Verification items for this drawing (mm, ordinates from the low corner). A direction names the side the tool comes from. Coordinates: 2 decimals unless noted, no trailing zeros. Write each loop counter-clockwise with the first axis right and the second up, starting at its lowest first coordinate (ties: lowest second). Pieces come first, ordered by that corner, then holes. Notation, with made-up numbers: M 86.25,-15.75 L 98.25,-15.75 A7 ccw 98.25,-4.75 Z; hole C 89,-5.75 d11. An arc over 180 degrees is marked long. Write each question's results on one line, items separated by ' | '.
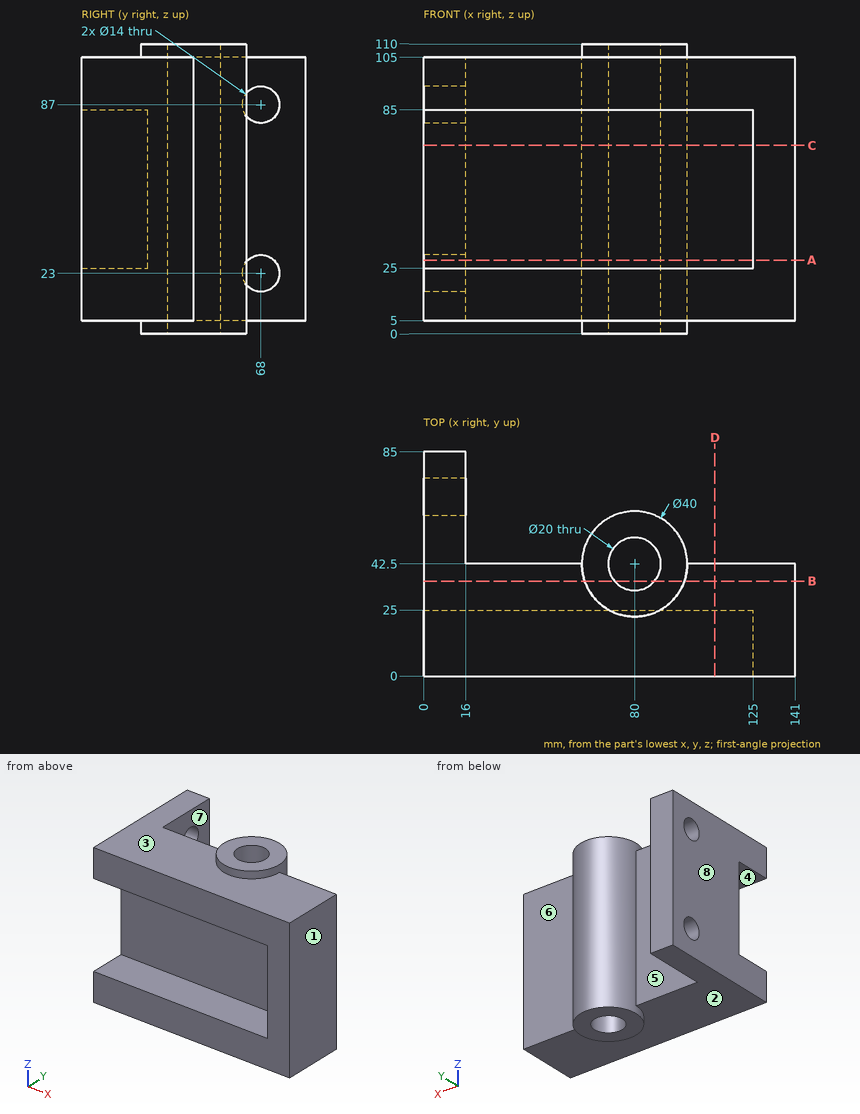
Q1. Sectioned sample at C-C on z = 71.5. Record the cut outline in (x, y).
Geometry check:
outline: M 0,25 L 125,25 L 125,0 L 141,0 L 141,42.5 L 100,42.5 A20 ccw 60,42.5 L 16,42.5 L 16,85 L 0,85 Z; hole C 80,42.5 d20
Q2. Scan lines: probe 1 along Z at (x, y) = (9.5, 68); probe 2 along Z at (x, y) = (91.5, 9.5); probe 3 along X at (y, z) = (48, 102). Record each from-to range of solid material in increasing order.
Geometry check:
probe 1: z = 5 to 16, 30 to 80, 94 to 105 | probe 2: z = 5 to 25, 85 to 105 | probe 3: x = 0 to 16, 60.77 to 71.65, 88.35 to 99.23
Q3. Access from +Z, -Z, +X, -X, +Y, -Y to the whole of each face (thin tool, end or side, straight path). Record for the marked faces 1, 2, 3, 4 and 5.
Geometry check:
face 1: +Z, -Z, +X, +Y, -Y | face 2: -Z, -Y | face 3: +Z, -Y | face 4: -X, -Y | face 5: +Z, -Z, +Y
Q4. Depth check by flat-ended pin: P1, Ø20, axis at x = 35, y = 9.5, coming from the +Z side; P2, Ø8, axis at x = 80.5, z = 50.5, coming from the -Y side; P3, Ø2, axis at x = 68.5, y = 20, coming from the -Z side; P4, Ø8.5, axis at y = 68, z = 23, coming from the +X side. Enter the tip coordinate at first touch or a pass-through.
Geometry check:
P1: stops at z = 105 | P2: stops at y = 25 | P3: stops at z = 5 | P4: passes through
Q5. Sectioned sample at A-A on z = 28. Record the cut outline in (x, y).
Geometry check:
outline: M 0,25 L 125,25 L 125,0 L 141,0 L 141,42.5 L 100,42.5 A20 ccw 60,42.5 L 16,42.5 L 16,63.1 L 0,63.1 Z; M 0,72.9 L 16,72.9 L 16,85 L 0,85 Z; hole C 80,42.5 d20
Q6. Mould release check, pull along X, two halves, no side actions. Record for the marked faces 6, 7 and 8: pulls with the +X half, pulls with the -X half, needs draft (parallel to the pull), parting line crosses it, or undercut.
Geometry check:
face 6: needs draft | face 7: undercut | face 8: pulls with the -X half
Q7. Sectioned sample at D-D on x = 110.5. Record the cut outline in (y, z).
Geometry check:
outline: M 0,5 L 42.5,5 L 42.5,105 L 0,105 L 0,85 L 25,85 L 25,25 L 0,25 Z
Q8. Sectioned sample at B-B on y = 36. Record the cut outline in (x, z), and give its area (3 significant figures).
Geometry check:
outline: M 0,5 L 61.09,5 L 61.09,0 L 72.4,0 L 72.4,110 L 61.09,110 L 61.09,105 L 0,105 Z; M 87.6,0 L 98.91,0 L 98.91,5 L 141,5 L 141,105 L 98.91,105 L 98.91,110 L 87.6,110 Z | area: 12,800 mm2
